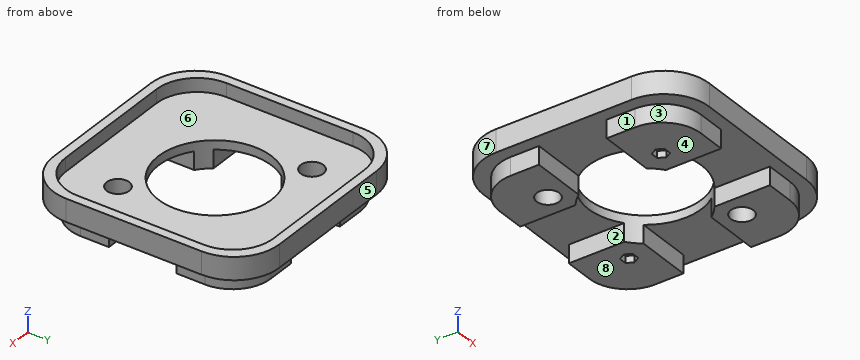
from build123d import *

# Parameters (mm, degrees)
BOX_W           = 30
BOX_H           = 100
BOX_DEPTH       = 10
BOX001_W        = 100
BOX001_H        = 30
BOX001_DEPTH    = 10
CYLINDER_R      = 25
CYLINDER_DEPTH  = 22
PAD_DEPTH       = 10
PAD001_DEPTH    = 18
POCKET_DEPTH    = 6
POCKET001_DEPTH = 3
COPYSKETCH005_R = 5
POCKET002_DEPTH = 18.001


with BuildPart() as cubo:
    # Box → Box (new body)
    with BuildSketch(Plane(origin=(-15, -50, -10), x_dir=(1, 0, 0), z_dir=(0, 0, 1))):
        with Locations((15, 50)):
            Rectangle(BOX_W, BOX_H)
    extrude(amount=BOX_DEPTH)


with BuildPart() as cubo001:
    # Box001 → Box001 (new body)
    with BuildSketch(Plane(origin=(-50, -15, -10), x_dir=(1, 0, 0), z_dir=(0, 0, 1))):
        with Locations((50, 15)):
            Rectangle(BOX001_W, BOX001_H)
    extrude(amount=BOX001_DEPTH)


with BuildPart() as fusion:
    # Cylinder → Cylinder (new body)
    with BuildSketch(Plane.XY.offset(-10)):
        Circle(CYLINDER_R)
    extrude(amount=CYLINDER_DEPTH)

    # Fusion: union Cubo, Cubo001
    add(cubo.part)
    add(cubo001.part)


with BuildPart() as cut:
    # Sketch → Pad (new body)
    with BuildSketch(Plane.XY):
        with BuildLine():
            Line((-30, 50), (30, 50))
            ThreePointArc((50, 30), (44.142136, 44.142136), (30, 50))
            Line((50, 30), (50, -30))
            ThreePointArc((30, -50), (44.142136, -44.142136), (50, -30))
            Line((30, -50), (-30, -50))
            ThreePointArc((-50, -30), (-44.142136, -44.142136), (-30, -50))
            Line((-50, -30), (-50, 30))
            ThreePointArc((-30, 50), (-44.142136, 44.142136), (-50, 30))
        make_face()
    extrude(amount=PAD_DEPTH)

    # Sketch001 (on Face10 of Pad) → Pad001 (join)
    with BuildSketch(Plane.XY.offset(10)):
        with BuildLine():
            Line((-27.5, 44.5), (27.5, 44.5))
            ThreePointArc((44.5, 27.5), (39.520815, 39.520815), (27.5, 44.5))
            Line((44.5, 27.5), (44.5, -27.5))
            ThreePointArc((27.5, -44.5), (39.520815, -39.520815), (44.5, -27.5))
            Line((27.5, -44.5), (-27.5, -44.5))
            ThreePointArc((-44.5, -27.5), (-39.520815, -39.520815), (-27.5, -44.5))
            Line((-44.5, -27.5), (-44.5, 27.5))
            ThreePointArc((-27.5, 44.5), (-39.520815, 39.520815), (-44.5, 27.5))
        make_face()
    extrude(amount=-PAD001_DEPTH)

    # CopySketch003 → Pocket (cut)
    with BuildSketch(Plane.XY.offset(10)):
        with BuildLine():
            Line((-28, 46), (28, 46))
            ThreePointArc((46, 28), (40.727922, 40.727922), (28, 46))
            Line((46, 28), (46, -28))
            ThreePointArc((28, -46), (40.727922, -40.727922), (46, -28))
            Line((28, -46), (-28, -46))
            ThreePointArc((-46, -28), (-40.727922, -40.727922), (-28, -46))
            Line((-46, -28), (-46, 28))
            ThreePointArc((-28, 46), (-40.727922, 40.727922), (-46, 28))
        make_face()
    extrude(amount=-POCKET_DEPTH, mode=Mode.SUBTRACT)

    # Sketch002 (on Face27 of Pocket) → Pocket001 (cut)
    with BuildSketch(Plane(origin=(0, 0, -8), x_dir=(1, 0, 0), z_dir=(0, 0, -1))):
        Polygon((-23.35, 22.142116), (-21.7, 25), (-23.35, 27.857884), (-26.65, 27.857884), (-28.3, 25), (-26.65, 22.142116), align=None)
        Polygon((28.3, -25), (26.65, -22.142116), (23.35, -22.142116), (21.7, -25), (23.35, -27.857884), (26.65, -27.857884), align=None)
    extrude(amount=-POCKET001_DEPTH, mode=Mode.SUBTRACT)

    # CopySketch005 → Pocket002 (cut, through all)
    with BuildSketch(Plane(origin=(0, 0, -8), x_dir=(1, 0, 0), z_dir=(0, 0, -1))):
        with Locations((25, 25)):
            Circle(COPYSKETCH005_R)
        with Locations((-25, -25)):
            Circle(COPYSKETCH005_R)
    extrude(amount=-POCKET002_DEPTH, mode=Mode.SUBTRACT)

    # Cut: cut Fusion
    add(fusion.part, mode=Mode.SUBTRACT)


solid = cut.part
Geometry: final body of the model. Coordinates: model frame, mm. Face numbers are marked on the shaded views. A direction names the side the tool comes from. Give positions to 0.01 mm unless a question says otherwise; leave off trailing zeros. Loops run counter-clockwise (first coordinate to the right, second up) from the corner with the lowest first, then second, coordinate; pieces in that order, holes last. Notation, with made-up numbers: M 62.5,-35.5 L 83.5,-35.5 A11 cw 83.5,-28.5 Z; hole C 23.5,43.5 d2. An arc over 180 degrees is marked long. Put each result on its own line as item: value.
1) Cut plane A-A, the plane z = -3.25. Return the cut outline in (x, y), plus the area to 3 significant figures.
Computed values:
outline: M -44.5,-27.5 A17 ccw -27.5,-44.5 L -15,-44.5 L -15,-20 A25 cw -20,-15 L -44.5,-15 Z; M -44.5,15 L -20,15 A25 cw -15,20 L -15,44.5 L -27.5,44.5 A17 ccw -44.5,27.5 Z; M 15,-44.5 L 27.5,-44.5 A17 ccw 44.5,-27.5 L 44.5,-15 L 20,-15 A25 cw 15,-20 Z; M 15,20 A25 cw 20,15 L 44.5,15 L 44.5,27.5 A17 ccw 27.5,44.5 L 15,44.5 Z; hole C -25,25 d10; hole C 25,-25 d10
area: 3,020 mm^2
2) Cut plane B-B, the plane x = 0. Return the cut outline in (y, z).
Computed values:
outline: M -50,0 L -25,0 L -25,4 L -46,4 L -46,10 L -50,10 Z; M 25,0 L 50,0 L 50,10 L 46,10 L 46,4 L 25,4 Z
3) Cut plane D-D, the plane z = 7.5. Return the cut outline in (x, y), plus the area to 3 significant figures.
Computed values:
outline: M -50,-30 A20 ccw -30,-50 L 30,-50 A20 ccw 50,-30 L 50,30 A20 ccw 30,50 L -30,50 A20 ccw -50,30 Z; hole M -46,-28 A18 ccw -28,-46 L 28,-46 A18 ccw 46,-28 L 46,28 A18 ccw 28,46 L -28,46 A18 ccw -46,28 Z
area: 1,470 mm^2
4) First-contact query: P1, Ø13, axis at x = 25, y = -25, coming from the +Z side; P2, Ø4, axis at y = -33, z = -2.5, coming from the -X side; P3, Ø9, axis at x = -34, z = -3.5, coming from the +Y side; P4, Ø5, axis at y = -11.5, z = -4, coming from the -X side. Flat tips, straight axial feed; report the tip coordinate or a pass-through.
Computed values:
P1: stops at z = 4
P2: stops at x = -44.14
P3: stops at y = 49.97
P4: passes through
5) Mould query, pull axis X, two halves, no side actions, for the marked faces 6, 7 and 8. Classes: released by +X, released by -X, zero draft, split by the parting line, or undercut.
Computed values:
face 6: undercut
face 7: released by -X
face 8: zero draft
6) Reachability of the marked faces 1, 2, 3, 4 and 5 from +Z, -Z, +X, -X, +Y, -Y: full face, straight path, thin tool, end or side. Return the list, or none.
Computed values:
face 1: -Z, -X, +Y, -Y
face 2: -Z, +Y, -Y
face 3: -Z, -X, -Y
face 4: -Z, +X, -X, +Y, -Y
face 5: +Z, -Z, +X, -X, +Y
7) Material intervals for L1, parallel to X at y = 25, z = -0.25; L2, parallel to Y at x = -25, z = -4.5; L3, parallel to Y at x = 22, z = 4.25, sorted ascending. Write a range as from..to.
Computed values:
L1: x = -44.5..-30, -20..-15, 15..44.5
L2: y = -44.5..-15, 15..20, 30..44.5
L3: y = -50..-46, 46..50
